The model under review builds one solid part; all positions refer to its coordinate system, in mm. A direction names the side the tool comes from. Round coordinates to 2 decimals unless told otherwise and drop trailing zeros. Write each loop counter-clockwise with the first axis right and the second up, starting at its lowest first coordinate (ties: lowest second). Pieces come first, ordered by that corner, then holes. Notation, with made-up numbers: (5.25, 26) -> (41.25, 26) arc R32 cw to (41.25, 57) -> close; hole circle Ø2 at (8.25, 26). An arc over 180 degrees is marked (long way). Return JSON: item names as keys, results as strings. Group by question number.
1. Clearance check with flat-ended pins moving along their axes: P1, Ø12, axis at x = 102, y = -2.5, coming from the -Z side; P2, Ø2, axis at x = 34, y = -6, coming from the -Z side; P3, Ø4, axis at x = 97, z = -9, coming from the -Y side. State where each tip first meets the part, or that it passes through.
2. Take a section at B-B, the plane x = 51. Write out the cut boundary in (y, z), then the cut area to 3 significant figures.
3. Mouldability with a two-part tool opening along Y and no side actions: class faces 3 (the flat face through (0, 8, 0)), 4 (the flat face through (62.611, 3.219, -5.474)), 5 (the cylindrical face through (62.61, -15.12, -11.59)), 6 (the flat face through (63, 6.35, 0)) as pulls with the +Y half, pulls with the -Y half, needs draft (parallel to the pull), parting line crosses it, or undercut.
4. Take a section at C-C, the plane y = 9.5. Write out the cut boundary in (x, z), then the cut area to 3 significant figures.
5. Take a section at D-D, the plane z = 14. Write out the cut boundary in (x, y), then the cut area to 3 significant figures.
6. Take a section at A-A, the plane z = 0. Write out the cut boundary in (x, y).
7. Tool access review of faces 1 (the flat face through (63, -6.35, 0)), 2 (the flat face through (127, 8, 0)): name each direction out of +Z, -Z, +X, -X, +Y, -Y from which nothing blocks a thin tool from reaching the whole face with its end or side.
8. For line 1 along Y through (x, z) = (120.5, 5); line 2 along Y through (x, z) = (102.5, 0.5); line 3 along Z through (x, y) = (23, 4.5), list the stretches that pass through material, from the lowest coordinate up. Write a range as from..to.
from build123d import *

# Parameters (mm, degrees)
F0_R     = 19.05
F1_DEPTH = 127


with BuildPart() as f1:
    # F0 (on Right) → F1 (new body)
    with BuildSketch(Plane.YZ):
        Circle(F0_R)
        Polygon((-6.35, 3.666174), (0, 7.332348), (6.35, 3.666174), (6.35, -3.666174), (0, -7.332348), (-6.35, -3.666174), align=None, mode=Mode.SUBTRACT)
    extrude(amount=F1_DEPTH)


solid = f1.part
Output:
{
 "1": {"P1": "stops at z = -19.05", "P2": "stops at z = -18.38", "P3": "stops at y = -17.72"},
 "2": {"outline": "circle Ø38.1 at (0, 0); hole (-6.35, -3.67) -> (0, -7.33) -> (6.35, -3.67) -> (6.35, 3.67) -> (0, 7.33) -> (-6.35, 3.67) -> close", "area": "1,000 mm^2"},
 "3": {"face 3": "needs draft", "face 4": "undercut", "face 5": "parting line crosses it", "face 6": "undercut"},
 "4": {"outline": "(0, -16.51) -> (127, -16.51) -> (127, 16.51) -> (0, 16.51) -> close", "area": "4,190 mm^2"},
 "5": {"outline": "(0, -12.92) -> (127, -12.92) -> (127, 12.92) -> (0, 12.92) -> close", "area": "3,280 mm^2"},
 "6": {"outline": "(0, -19.05) -> (127, -19.05) -> (127, -6.35) -> (0, -6.35) -> close; (0, 6.35) -> (127, 6.35) -> (127, 19.05) -> (0, 19.05) -> close"},
 "7": {"face 1": "+X, -X", "face 2": "+Z, -Z, +X, +Y, -Y"},
 "8": {"line 1": "y = -18.38..-4.04, 4.04..18.38", "line 2": "y = -19.04..-6.35, 6.35..19.04", "line 3": "z = -18.51..-4.73, 4.73..18.51"}
}
